Read the model definition and answer for the solid it produces. Units are mm, in the model's axes. Face numbers are marked on the shaded views. Coordinates: 2 decimals unless noted, no trailing zeros. Write each loop counter-clockwise with the first axis right and the second up, starting at its lowest first coordinate (ties: lowest second). Pieces come first, ordered by that corner, then holes. Notation, with made-up numbers: (48.25, -16) - (103.25, -16) arc R27 ccw to (103.25, 9) - close; hole circle Ø3 at (-22.75, 67). An arc over 180 degrees is marked (long way). Return JSON: item names as keys, results as strings.
```python
from build123d import *

# Parameters (mm, degrees)
SKETCH1_W              = 55.88
SKETCH1_H              = 25.4
SKETCH1_R              = 5.842
BOSS_EXTRUDE1_DEPTH    = 3.175
SKETCH2_R              = 2.54
CUT_EXTRUDE_4_40_DEPTH = 32.340965205
FILLET1_R              = 5.08


with BuildPart() as part:
    # Sketch1 → Boss-Extrude1 (new, symmetric)
    with BuildSketch(Plane.XY):
        Rectangle(SKETCH1_W, SKETCH1_H)
        Circle(SKETCH1_R, mode=Mode.SUBTRACT)
    extrude(amount=BOSS_EXTRUDE1_DEPTH, both=True)

    # Sketch2 → Cut-Extrude 4-40 (cut, through all)
    with BuildSketch(Plane.XY.offset(3.175)):
        with Locations((21.19, 0)):
            Circle(SKETCH2_R)
        with Locations(Location((-21.19, 0, 0), (0, 0, 180))):
            Circle(SKETCH2_R)
    extrude(amount=-CUT_EXTRUDE_4_40_DEPTH, mode=Mode.SUBTRACT)

    # Fillet1
    fillet1_edges = [part.edges().sort_by_distance(p)[0] for p in [
        (27.94, -12.7, 0),
        (-27.94, -12.7, 0),
        (-27.94, 12.7, 0),
        (27.94, 12.7, 0),
    ]]
    fillet(fillet1_edges, radius=FILLET1_R)


solid = part.part
```
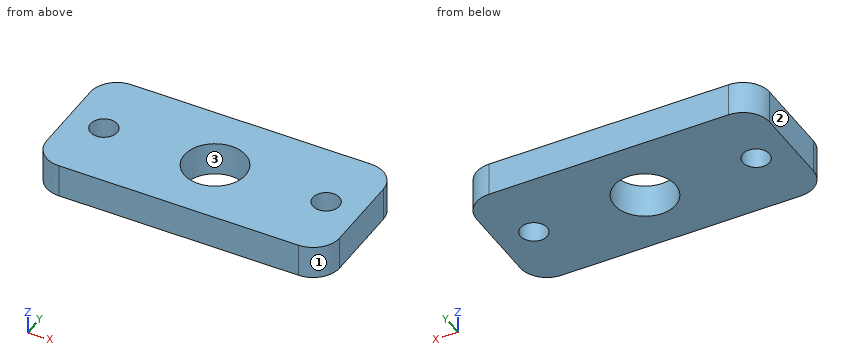
(1) A cutting plane is placed at B-B (y = 0). Determine the outline of the cut face in (x, z) (3 decimals).
Answer:
{"outline": "(-27.94, -3.175) - (-23.73, -3.175) - (-23.73, 3.175) - (-27.94, 3.175) - close; (-18.65, -3.175) - (-5.842, -3.175) - (-5.842, 3.175) - (-18.65, 3.175) - close; (5.842, -3.175) - (18.65, -3.175) - (18.65, 3.175) - (5.842, 3.175) - close; (23.73, -3.175) - (27.94, -3.175) - (27.94, 3.175) - (23.73, 3.175) - close"}
(2) A cutting plane is placed at D-D (y = 4.5). Determine the outline of the cut face in (x, z) (3 decimals), and give its area (3 significant figures).
Answer:
{"outline": "(-27.94, -3.175) - (-3.725, -3.175) - (-3.725, 3.175) - (-27.94, 3.175) - close; (3.725, -3.175) - (27.94, -3.175) - (27.94, 3.175) - (3.725, 3.175) - close", "area": "308 mm²"}
(3) A cutting plane is placed at C-C (z = 0.5). Determine the outline of the cut face in (x, y).
Answer:
{"outline": "(-27.94, -7.62) arc R5.08 ccw to (-22.86, -12.7) - (22.86, -12.7) arc R5.08 ccw to (27.94, -7.62) - (27.94, 7.62) arc R5.08 ccw to (22.86, 12.7) - (-22.86, 12.7) arc R5.08 ccw to (-27.94, 7.62) - close; hole circle Ø5.08 at (-21.19, 0); hole circle Ø11.68 at (0, 0); hole circle Ø5.08 at (21.19, 0)"}
(4) Straight lines are drawn through the part: line 1 (Y direction, x = 0, z = 1.5); line 2 (X direction, y = 1.75, z = -3); line 3 (Y direction, x = 21.19, z = -0.5). For each, find the intervals that lie inside material, in ascending order. Write a range as from..to.
Answer:
{"line 1": "-12.7..-5.84, 5.84..12.7", "line 2": "-27.94..-23.03, -19.35..-5.57, 5.57..19.35, 23.03..27.94", "line 3": "-12.7..-2.54, 2.54..12.7"}
(5) Determine the mould class of the marked faces 1, 2 and 3 for opening direction X: +X half, -X half, draft (parallel to the pull), parting line (faces both ways), or undercut.
Answer:
{"face 1": "+X half", "face 2": "-X half", "face 3": "undercut"}
(6) A cutting plane is placed at A-A (x = -21.19). Determine the outline of the cut face in (y, z) (3 decimals).
Answer:
{"outline": "(-12.7, -3.175) - (-2.54, -3.175) - (-2.54, 3.175) - (-12.7, 3.175) - close; (2.54, -3.175) - (12.7, -3.175) - (12.7, 3.175) - (2.54, 3.175) - close"}
